Autodesk Inventor part; units mm, degrees
ref_plane "YZ Plane" through (0, 0, 0) normal (1, 0, 0) x (0, 1, 0)
ref_plane "XZ Plane" through (0, 0, 0) normal (0, 1, 0) x (-1, 0, 0)
ref_plane "XY Plane" through (0, 0, 0) normal (0, 0, 1) x (1, 0, 0)
sketch "Sketch1" plane through (0, 0, 0) normal (0, 0, 1) x (1, 0, 0)
  circle A0 centre (-0.0091, 4.1481) radius 4.25
  point P0 (0, 0)
extrude "Extrusion1" add sketch "Sketch1" against normal blind 6.5
thread "Thread1"
sketch "Sketch2" plane through (-0.0091, 4.1481, 0) normal (0, 0, 1) x (1, 0, 0)
  line L0 (2.5727, -4.4349) -> (-2.5544, -4.4455)
  line L1 (-2.5544, -4.4455) -> (-5.1271, -0.0106)
  line L2 (-5.1271, -0.0106) -> (-2.5727, 4.4349)
  line L3 (-2.5727, 4.4349) -> (2.5544, 4.4455)
  line L4 (2.5544, 4.4455) -> (5.1271, 0.0106)
  line L5 (5.1271, 0.0106) -> (2.5727, -4.4349)
  point P0 (0.0091, -4.1481)
  point P1 (0, 0)
extrude "Extrusion2" add sketch "Sketch2" along normal blind 6.5
sketch "Sketch3" plane through (-0.0091, 4.1481, 6.5) normal (0, 0, 1) x (1, 0, 0)
  circle A0 centre (0, 0) radius 4.25
  point P0 (0.0091, -4.1481)
extrude "Extrusion3" add sketch "Sketch3" along normal blind 1.5
fillet "Fillet1" radius 1 1 edges at (-4.2591, 4.1481, 8)
sketch "Sketch4" plane through (-0.0091, 4.1481, 8) normal (0, 0, 1) x (1, 0, 0)
  circle A0 centre (0, 0) radius 3.25
  point P0 (0.0091, -4.1481)
extrude "Extrusion4" add sketch "Sketch4" along normal blind 1
sketch "Sketch5" plane through (-0.0091, 4.1481, 9) normal (0, 0, 1) x (1, 0, 0)
  point P0 (0.0091, -4.1481)
sketch "Sketch6" plane through (-0.0091, 4.1481, 9) normal (0, 0, 1) x (1, 0, 0)
  circle A0 centre (0, 0) radius 3.25
  circle A1 centre (0, 0) radius 2.5
  point P0 (0.0091, -4.1481)
  dimension "d11" = 5
extrude "Extrusion5" cut sketch "Sketch6" against normal through all contours A1
chamfer "Chamfer1" distance 1 angle 45 1 edges at (-4.2591, 4.1481, -6.5)
properties part number "Pushfit-Adapter"
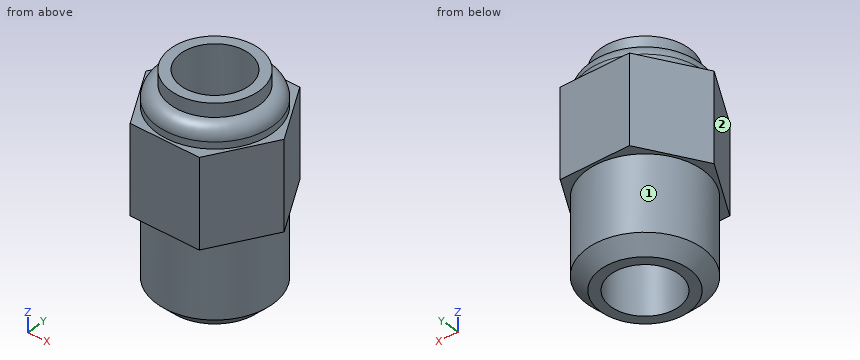
For this review, take the finished solid that the model builds, in its own axes (mm). Face numbers are marked on the shaded views. A direction names the side the tool comes from. Round coordinates to 2 decimals unless told otherwise and drop trailing zeros. Loops run counter-clockwise (first coordinate to the right, second up) from the corner with the lowest first, then second, coordinate; pieces in that order, holes last.
(1) Tool access review of the marked faces 1 and 2: name each direction out of +Z, -Z, +X, -X, +Y, -Y from which nothing blocks a thin tool from reaching the whole face with its end or side.
Returned:
face 1: -Z
face 2: +Z, -Z, -X, -Y
(2) Clearance check with flat-ended pins moving along their axes: P1, Ø3, axis at x = 2, y = 1, coming from the -Z side; P2, Ø1, axis at y = 1, z = 6, coming from the -X side; P3, Ø1.5, axis at y = 2, z = -2, coming from the -X side. State where each tip first meets the part, or that it passes through.
Returned:
P1: stops at z = -6.5
P2: stops at x = -3.61
P3: stops at x = -4.02
(3) We need section B-B (z = -4). Give the boundary of the cut face in (x, y), plus the area to 3 significant figures.
Returned:
outline: circle Ø8.5 at (-0.01, 4.15); hole circle Ø5 at (-0.01, 4.15)
area: 37.1 mm2
(4) We need section A-A (z = 4.25). Give the boundary of the cut face in (x, y), plus the area to 3 significant figures.
Returned:
outline: (-5.14, 4.14) - (-2.56, -0.3) - (2.56, -0.29) - (5.12, 4.16) - (2.55, 8.59) - (-2.58, 8.58) - close; hole circle Ø5 at (-0.01, 4.15)
area: 48.7 mm2
(5) Wall thickness on line 1 along X through (y, z) = (4.5, -2.75); line 2 along Y through (x, z) = (-2.25, -5.75); line 3 along Y through (x, z) = (-2, 3): over which ranges is each line inside the solid? List them lowest first.
Returned:
line 1: x = -4.24 to -2.48, 2.47 to 4.23
line 2: y = 0.83 to 3.04, 5.26 to 7.46
line 3: y = -0.3 to 2.64, 5.66 to 8.58
